from build123d import *

# Parameters (mm, degrees)
SKETCH2_R                  = 21
SKETCH2_W                  = 3.2
SKETCH2_H                  = 25.2
BOSS_EXTRUDE1_DEPTH        = 3
F_10_0_10_DIAMETER_HOLE1_D = 10
F_8_0_8_DIAMETER_HOLE1_D   = 8
F_12_0_12_DIAMETER_HOLE1_D = 12
CUT_EXTRUDE1_DEPTH         = 160.1679616
CUT_EXTRUDE1_DEPTH_BACK    = 160.1679616
F_6_0_6_DIAMETER_HOLE2_D   = 6
SKETCH27_R                 = 0.5
CUT_EXTRUDE2_DEPTH         = 160.1679616
FILLET1_R                  = 0.5


with BuildPart() as part:
    # Sketch2 → Boss-Extrude1 (new, symmetric)
    with BuildSketch(Plane.XY):
        Polygon((-68, 65), (95.2, 65), (110.2, 65), (110.2, -103), (0, -103), (-121.2, -103), (-121.2, 65), (-106.2, 65), align=None)
        Circle(SKETCH2_R, mode=Mode.SUBTRACT)
        with Locations((-77.6, 0)):
            Rectangle(SKETCH2_W, SKETCH2_H, mode=Mode.SUBTRACT)
        with Locations((66.6, 0)):
            Rectangle(SKETCH2_W, SKETCH2_H, mode=Mode.SUBTRACT)
    extrude(amount=BOSS_EXTRUDE1_DEPTH, both=True)

    # Ø10.0 (10) Diameter Hole1 (through all)
    with Locations(Plane.XY.offset(3)):
        with Locations((-68, 50), (-68, -55)):
            Hole(F_10_0_10_DIAMETER_HOLE1_D / 2)

    # Ø8.0 (8) Diameter Hole1 (through all)
    with Locations(Plane.XY.offset(3)):
        with Locations((-106.2, 50), (-106.2, -88), (95.2, -88), (95.2, 50)):
            Hole(F_8_0_8_DIAMETER_HOLE1_D / 2)

    # Ø12.0 (12) Diameter Hole1 (through all)
    with Locations(Plane(origin=(0, 0, -3), x_dir=(-1, 0, 0), z_dir=(0, 0, -1))):
        with Locations((-45, 0), (45, 0)):
            Hole(F_12_0_12_DIAMETER_HOLE1_D / 2)

    # Sketch18 → Cut-Extrude1 (cut, two sides: drawn at the far end of the back side and taken through both)
    with BuildSketch(Plane.XY.offset(3).offset(-CUT_EXTRUDE1_DEPTH_BACK)):
        with BuildLine():
            Line((-58.912310621, -25.006792223), (-61.673825181, -26.178985609))
            ThreePointArc((-61.673825181, -26.178985609), (2.922498953, -66.936230846), (63.720786592, -20.704138623))
            Line((63.720786592, -20.704138623), (60.867617043, -19.77708764))
            ThreePointArc((60.867617043, -19.77708764), (2.791640791, -63.939086181), (-58.912310621, -25.006792223))
        make_face()
    extrude(amount=CUT_EXTRUDE1_DEPTH + CUT_EXTRUDE1_DEPTH_BACK, mode=Mode.SUBTRACT)

    # Ø6.0 (6) Diameter Hole2 (through all)
    with Locations(Plane(origin=(0, 0, -3), x_dir=(-1, 0, 0), z_dir=(0, 0, -1))):
        with Locations((49, -61), (-52, -61)):
            Hole(F_6_0_6_DIAMETER_HOLE2_D / 2)

    # Sketch27 → Cut-Extrude2 (cut, through all)
    with BuildSketch(Plane(origin=(0, 0, -3), x_dir=(-1, 0, 0), z_dir=(0, 0, -1))):
        with Locations((-65, 12.6)):
            Circle(SKETCH27_R)
        with Locations((-68.2, 12.6)):
            Circle(SKETCH27_R)
        with Locations((-65, -12.6)):
            Circle(SKETCH27_R)
        with Locations((-68.2, -12.6)):
            Circle(SKETCH27_R)
        with Locations((79.2, 12.6)):
            Circle(SKETCH27_R)
        with Locations((76, 12.6)):
            Circle(SKETCH27_R)
        with Locations((79.2, -12.6)):
            Circle(SKETCH27_R)
        with Locations((76, -12.6)):
            Circle(SKETCH27_R)
    extrude(amount=-CUT_EXTRUDE2_DEPTH, mode=Mode.SUBTRACT)

    # Fillet1
    fillet1_edges = [part.edges().sort_by_distance(p)[0] for p in [
        (68.2, 12.1, 0),
        (68.2, -12.1, 0),
        (65.5, -12.6, 0),
        (65, 12.1, 0),
        (-76, 12.1, 0),
        (-76, -12.1, 0),
        (-78.7, -12.6, 0),
        (-79.2, 12.1, 0),
        (-78.7, 12.6, 0),
        (67.7, -12.6, 0),
        (65, -12.1, 0),
        (67.7, 12.6, 0),
        (-76.5, -12.6, 0),
        (-79.2, -12.1, 0),
        (-76.5, 12.6, 0),
        (65.5, 12.6, 0),
    ]]
    fillet(fillet1_edges, radius=FILLET1_R)


solid = part.part
Geometry: final body of the model. Coordinates: model frame, mm. A direction names the side the tool comes from. Give positions to 0.01 mm unless a question says otherwise; leave off trailing zeros. Write each loop counter-clockwise with the first axis right and the second up, starting at its lowest first coordinate (ties: lowest second). Pieces come first, ordered by that corner, then holes. Notation, with made-up numbers: M 76.25,-24.5 L 115.25,-24.5 A22 ccw 115.25,4.5 Z; hole C -27.5,-7 d6. An arc over 180 degrees is marked long. Answer in a Markdown table with one row per item. Add a question column.
(1) Section D-D on x = 25. Return loops of the section in (y, z).
(2) Section A-A on x = -68. Return loops of the section in (y, z), and give its area (3 significant figures).
(3) Section C-C on y = 0. Return loops of the section in (x, z).
(4) Reachability of faces 5 (the flat face through (-4, -36, 3)), 6 (the flat face through (-76, 0, 0)) from +Z, -Z, +X, -X, +Y, -Y: full face, straight path, thin tool, end or side. Return the list, or none.
(5) Mould query, pull axis X, two halves, no side actions, for faces 1 (the flat face through (-79.2, 0, 0)), 2 (the cylindrical face through (-102.204, 50.176, -0.042)), 3 (the flat face through (110.2, -18, 0)), 4 (the flat face through (-4, 65, 0)). Classes: +X half, -X half, draft (parallel to the pull), parting line (faces both ways), or undercut.
(6) Ray query, line 1 (Y direction, x = 95.2, z = -1.6); line 2 (Y direction, x = 16, z = 1.45); line 3 (X direction, y = -12, z = -2.1). Return the intervals inside material, ascending.
(7) Section B-B on y = -88. Return loops of the section in (x, z), and give its area (3 significant figures).
Result set:
| question | item | result |
|---|---|---|
| 1 | outline | M -103,-3 L -62.16,-3 L -62.16,3 L -103,3 Z; M -58.92,-3 L 65,-3 L 65,3 L -58.92,3 Z |
| 2 | outline | M -103,-3 L -60,-3 L -60,3 L -103,3 Z; M -50,-3 L 45,-3 L 45,3 L -50,3 Z; M 55,-3 L 65,-3 L 65,3 L 55,3 Z |
| 2 | area | 888 mm^2 |
| 3 | outline | M -121.2,-3 L -79.2,-3 L -79.2,3 L -121.2,3 Z; M -76,-3 L -51,-3 L -51,3 L -76,3 Z; M -39,-3 L -21,-3 L -21,3 L -39,3 Z; M 21,-3 L 39,-3 L 39,3 L 21,3 Z; M 51,-3 L 65,-3 L 65,3 L 51,3 Z; M 68.2,-3 L 110.2,-3 L 110.2,3 L 68.2,3 Z |
| 4 | face 5 | +Z, +X, -X, +Y, -Y |
| 4 | face 6 | +Z, -Z |
| 5 | face 1 | undercut |
| 5 | face 2 | undercut |
| 5 | face 3 | +X half |
| 5 | face 4 | draft |
| 6 | line 1 | y = -103 to -92, -84 to 46, 54 to 65 |
| 6 | line 2 | y = -103 to -65.06, -61.97 to -13.6, 13.6 to 65 |
| 6 | line 3 | x = -121.2 to -79.28, -75.92 to -17.23, 17.23 to 64.92, 68.28 to 110.2 |
| 7 | outline | M -121.2,-3 L -110.2,-3 L -110.2,3 L -121.2,3 Z; M -102.2,-3 L 91.2,-3 L 91.2,3 L -102.2,3 Z; M 99.2,-3 L 110.2,-3 L 110.2,3 L 99.2,3 Z |
| 7 | area | 1,290 mm^2 |
